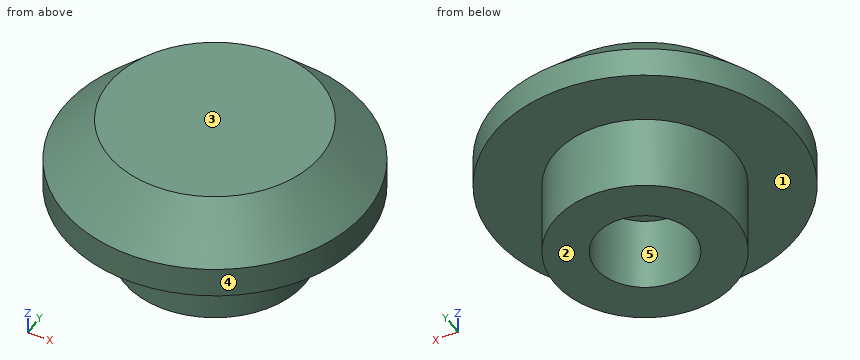
```python
from build123d import *

# Parameters (mm, degrees)
BOSS_EXTRUDE1_DEPTH      = 5
BOSS_EXTRUDE1_DEPTH_BACK = 5
SKETCH1_R                = 6
SKETCH1_R_2              = 3.25
SKETCH2_R                = 10.000000149
BOSS_EXTRUDE2_DEPTH      = 5
CHAMFER1_SIZE            = 3


with BuildPart() as part:
    # Sketch1 → Boss-Extrude1 (new, two sides: drawn at the far end of the back side and taken through both)
    with BuildSketch(Plane.XY.offset(-BOSS_EXTRUDE1_DEPTH_BACK)):
        Circle(SKETCH1_R)
        Circle(SKETCH1_R_2, mode=Mode.SUBTRACT)
    extrude(amount=BOSS_EXTRUDE1_DEPTH + BOSS_EXTRUDE1_DEPTH_BACK)

    # Sketch2 → Boss-Extrude2 (add)
    with BuildSketch(Plane.XY):
        Circle(SKETCH2_R)
    extrude(amount=BOSS_EXTRUDE2_DEPTH)

    # Chamfer1
    chamfer1_edges = [part.edges().sort_by_distance(p)[0] for p in [
        (-10.000000149, 0, 5),
    ]]
    chamfer(chamfer1_edges, length=CHAMFER1_SIZE)


solid = part.part
```
For this review, take the finished solid that the model builds, in its own axes (mm). Face numbers are marked on the shaded views. A direction names the side the tool comes from. Round coordinates to 2 decimals unless told otherwise and drop trailing zeros. Loops run counter-clockwise (first coordinate to the right, second up) from the corner with the lowest first, then second, coordinate; pieces in that order, holes last.
Q1. Insertion check: pin 1 Ø3 at (x, z) = (-5.5, -1) entering from +Y; pin 2 Ø3 at (y, z) = (-2, 3) entering from +X; pin 3 Ø3 at (x, z) = (-3, 3.5) entering from -Y. Each pin has a flat end and moves straight along its axis. Give the tip position at first contact, or say it passes through.
Result sheet:
pin 1: stops at y = 8.99
pin 2: stops at x = 9.96
pin 3: stops at y = -9.6
Q2. To check wall thickness, follow line 1 along X through (y, z) = (0, -4); line 2 along Z through (x, y) = (-2, 6.25). State the ranges of each line that lie inside material, in increasing order.
Result sheet:
line 1: x = -6 to -3.25, 3.25 to 6
line 2: z = 0 to 5
Q3. Add section D-D on z = 3.25. Write out the cut boundary in (x, y).
Result sheet:
outline: circle Ø17.5 at (0, 0)
Q4. Add section C-C on z = -3. Write out the cut boundary in (x, y).
Result sheet:
outline: circle Ø12 at (0, 0); hole circle Ø6.5 at (0, 0)
Q5. Add section A-A on y = 0. Write out the cut boundary in (x, z).
Result sheet:
outline: (-10, 0) - (-6, 0) - (-6, -5) - (-3.25, -5) - (-3.25, 0) - (3.25, 0) - (3.25, -5) - (6, -5) - (6, 0) - (10, 0) - (10, 2) - (7, 5) - (-7, 5) - (-10, 2) - close
Q6. Mouldability with a two-part tool opening along Y and no side actions: class the marked faces 3, 4 and 5 as +Y half, -Y half, draft (parallel to the pull), parting line (faces both ways), or undercut.
Result sheet:
face 3: draft
face 4: parting line
face 5: undercut
Q7. Machinability: for the marked faces 1 and 2, which of the approach directions +Z, -Z, +X, -X, +Y, -Y give a long, thin tool a straight path to every point of the face, cutting with its end or side? Answer none if there is none.
Result sheet:
face 1: -Z
face 2: -Z, +X, -X, +Y, -Y
